Model file for the job. Use its own axes, mm. A direction names the side the tool comes from. Round coordinates to 2 decimals unless told otherwise and drop trailing zeros. Loops run counter-clockwise (first coordinate to the right, second up) from the corner with the lowest first, then second, coordinate; pieces in that order, holes last. Notation, with made-up numbers: M 60,-7 L 115,-7 A7 cw 115,4 Z; hole C 70.5,-28 d7. An arc over 180 degrees is marked long. Use a Markdown table: item, result. Add a question column.
Q1. Cut at A-A (x = 0). Give the cut face in (y, z).
Q2. Cut at C-C (y = 0.15). Give the cut face in (x, z) (3 decimals), plus the area to 3 significant figures.
Q3. Mould opens along Z. For faces 1 (the face through (0, 0, -12.601)), 2 (the face through (2.5, 0, -10)), 3 (the face through (-1.678, -0.01, -6.393)) say: +Z half, -Z half, draft (parallel to the pull), parting line (faces both ways), or undercut.
Q4. Tool access for faces 4 (the face through (1.678, -0.01, 6.393)), 5 (the face through (-1.694, -0.01, 6.431)), 6 (the face through (0.672, 0.01, -8.946)): list every direction of +Z, -Z, +X, -X, +Y, -Y with a clear straight run to the whole face (end or side of a thin tool).
Q5. Cut at D-D (x = -2.1). Give the cut face in (y, z).
Q6. Cut at B-B (z = 10). Give the cut face in (x, y).
Q7. Probe line 1 (Z direction, x = 0, y = 0.4); line 2 (X direction, y = -0.6, z = -4); line 3 (Z direction, x = 2.1, y = -0.6). List the from-to ranges inside material, lowest first. Write a range as from..to.
from build123d import *

# Parameters (mm, degrees)
F1_R     = 1.25
F2_DEPTH = 0.75


with BuildPart() as f2:
    # F1 (on Front) → F2 (new body, symmetric)
    with BuildSketch(Plane.XZ):
        with BuildLine():
            ThreePointArc((0.75, 0), (0.9196994782, 0.8062257748), (1.4, 1.4756354563))
            Line((1.4, 1.4756354563), (1.4, 5))
            ThreePointArc((1.4, 5), (1.6863063932, 6.4120021246), (2.5, 7.6009613607))
            Line((2.5, 7.6009613607), (2.5, 12.6009613607))
            Line((2.5, 12.6009613607), (0, 12.6009613607))
            Line((0, 12.6009613607), (-2.5, 12.6009613607))
            Line((-2.5, 12.6009613607), (-2.5, 7.6009613607))
            ThreePointArc((-2.5, 7.6009613607), (-1.6863063932, 6.4120021246), (-1.4, 5))
            Line((-1.4, 5), (-1.4, 1.4756354563))
            ThreePointArc((-1.4, 1.4756354563), (-0.9196994782, 0.8062257748), (-0.75, 0))
            ThreePointArc((-0.75, 0), (-0.9196994782, -0.8062257748), (-1.4, -1.4756354563))
            Line((-1.4, -1.4756354563), (-1.4, -5))
            ThreePointArc((-1.4, -5), (-1.6863063932, -6.4120021246), (-2.5, -7.6009613607))
            Line((-2.5, -7.6009613607), (-2.5, -12.6009613607))
            Line((-2.5, -12.6009613607), (0, -12.6009613607))
            Line((0, -12.6009613607), (2.5, -12.6009613607))
            Line((2.5, -12.6009613607), (2.5, -7.6009613607))
            ThreePointArc((2.5, -7.6009613607), (1.6863063932, -6.4120021246), (1.4, -5))
            Line((1.4, -5), (1.4, -1.4756354563))
            ThreePointArc((1.4, -1.4756354563), (0.9196994782, -0.8062257748), (0.75, 0))
        make_face()
        with Locations((0, -10)):
            Circle(F1_R, mode=Mode.SUBTRACT)
        with Locations((0, 10)):
            Circle(F1_R, mode=Mode.SUBTRACT)
    extrude(amount=F2_DEPTH, both=True)


solid = f2.part
Checked values:
| question | item | result |
|---|---|---|
| 1 | outline | M -0.75,-12.6 L 0.75,-12.6 L 0.75,-11.25 L -0.75,-11.25 Z; M -0.75,-8.75 L 0.75,-8.75 L 0.75,8.75 L -0.75,8.75 Z; M -0.75,11.25 L 0.75,11.25 L 0.75,12.6 L -0.75,12.6 Z |
| 2 | outline | M -2.5,-12.601 L 2.5,-12.601 L 2.5,-7.601 A3.625 cw 1.4,-5 L 1.4,-1.476 A2 cw 1.4,1.476 L 1.4,5 A3.625 cw 2.5,7.601 L 2.5,12.601 L -2.5,12.601 L -2.5,7.601 A3.625 cw -1.4,5 L -1.4,1.476 A2 cw -1.4,-1.476 L -1.4,-5 A3.625 cw -2.5,-7.601 Z; hole C 0,-10 d2.5; hole C 0,10 d2.5 |
| 2 | area | 83.6 mm^2 |
| 3 | face 1 | -Z half |
| 3 | face 2 | draft |
| 3 | face 3 | undercut |
| 4 | face 4 | +X, +Y, -Y |
| 4 | face 5 | -X, +Y, -Y |
| 4 | face 6 | +Y, -Y |
| 5 | outline | M -0.75,-12.6 L 0.75,-12.6 L 0.75,-7.14 L -0.75,-7.14 Z; M -0.75,7.14 L 0.75,7.14 L 0.75,12.6 L -0.75,12.6 Z |
| 6 | outline | M -2.5,-0.75 L -1.25,-0.75 L -1.25,0.75 L -2.5,0.75 Z; M 1.25,-0.75 L 2.5,-0.75 L 2.5,0.75 L 1.25,0.75 Z |
| 7 | line 1 | z = -12.6..-11.25, -8.75..8.75, 11.25..12.6 |
| 7 | line 2 | x = -1.4..1.4 |
| 7 | line 3 | z = -12.6..-7.14, 7.14..12.6 |
